from build123d import *

# Parameters (mm, degrees)
F0_W      = 858
F0_H      = 170
F1_DEPTH  = 19
F2_W      = 19
F2_H      = 170
F3_DEPTH  = 590
F4_W      = 19
F4_H      = 170
F5_DEPTH  = 824
F6_W      = 820
F6_H      = 5
F7_DEPTH  = 8
F8_W      = 820
F8_H      = 5
F9_DEPTH  = 8
F11_DEPTH = 8
F13_DEPTH = 8
F14_R     = 2
F15_DEPTH = 19


with BuildPart() as f1:
    # F0 (on Front) → F1 (new body)
    with BuildSketch(Plane.XZ):
        with Locations((-9.432035, -4.196442)):
            Rectangle(F0_W, F0_H)
    extrude(amount=F1_DEPTH)

    # F2 (on face) → F3 (join)
    with BuildSketch(Plane(origin=(0, 0, 0), x_dir=(-1, 0, 0), z_dir=(0, 1, 0))):
        with Locations((-410.067965, -4.196442)):
            Rectangle(F2_W, F2_H)
        with Locations((428.932035, -4.196442)):
            Rectangle(F2_W, F2_H)
    extrude(amount=F3_DEPTH)

    # F4 (on face) → F5 (join)
    with BuildSketch(Plane(origin=(400.567965, 0, 0), x_dir=(0, -1, 0), z_dir=(-1, 0, 0))):
        with Locations((-580.5, -4.196442)):
            Rectangle(F4_W, F4_H)
    extrude(amount=F5_DEPTH)

    # F6 (on face) → F7 (cut)
    with BuildSketch(Plane.XZ.offset(-571)):
        with Locations((-9.432035, -81.696442)):
            Rectangle(F6_W, F6_H)
    extrude(amount=-F7_DEPTH, mode=Mode.SUBTRACT)

    # F8 (on face) → F9 (cut)
    with BuildSketch(Plane(origin=(0, 0, 0), x_dir=(-1, 0, 0), z_dir=(0, 1, 0))):
        with Locations((9.432035, -81.696442)):
            Rectangle(F8_W, F8_H)
    extrude(amount=-F9_DEPTH, mode=Mode.SUBTRACT)

    # F10 (on face) → F11 (cut)
    with BuildSketch(Plane.YZ.offset(-419.432035)):
        Polygon((0, -79.196442), (-8, -79.196442), (-8, -84.196442), (0, -84.196442), (571, -84.196442), (579, -84.196442), (579, -79.196442), (571, -79.196442), align=None)
    extrude(amount=-F11_DEPTH, mode=Mode.SUBTRACT)

    # F12 (on face) → F13 (cut)
    with BuildSketch(Plane(origin=(400.567965, 0, 0), x_dir=(0, -1, 0), z_dir=(-1, 0, 0))):
        Polygon((8, -84.196442), (8, -79.196442), (0, -79.196442), (-571, -79.196442), (-579, -79.196442), (-579, -84.196442), (-571, -84.196442), (0, -84.196442), align=None)
    extrude(amount=-F13_DEPTH, mode=Mode.SUBTRACT)

    # F14 (on face) → F15 (cut)
    with BuildSketch(Plane.XZ.offset(19)):
        Circle(F14_R)
    extrude(amount=-F15_DEPTH, mode=Mode.SUBTRACT)


solid = f1.part
Model file for the job. Use its own axes, mm. A direction names the side the tool comes from. Coordinates: 2 decimals unless noted, no trailing zeros. Write each loop counter-clockwise with the first axis right and the second up, starting at its lowest first coordinate (ties: lowest second). Pieces come first, ordered by that corner, then holes. Notation, with made-up numbers: (-20, -2.5) -> (-12, -2.5) arc R18 cw to (-12, 19.5) -> close; hole circle Ø8 at (67, 59). An arc over 180 degrees is marked (long way). One line per item, written item: value. Start each with the question number.
1) Slice it at B-B on x = -40. Write the cut outline in (y, z), then the cut area to 3 significant figures.
2) Probe probe 1 along Y at (x, z) = (-234, 69.5); probe 2 along Z at (x, y) = (0, -6); probe 3 along Z at (x, y) = (0, -14). List the from-to ranges inside material, lowest first.
3) Pull direction Y, two halves, no side cores. Call faces 3 (the face through (-438.432, 290, -5)), 4 (the face through (-3, 590, -5)), 5 (the face through (-419.432, 282, 0)), 6 (the face through (-4, 571, 0)): +Y half, -Y half, draft (parallel to the pull), parting line (faces both ways), or undercut.
4) Flat gauge pin, fed straight in: pin 1 Ø4.5 at (x, z) = (0, 0) entering from -Y. Where does the tip first touch, or does it go through?
5) Which spindle directions (+Z, -Z, +X, -X, +Y, -Y) get a long thin tool onto all of the face, cutting with end or side? Do faces 1 (the face through (-15, -19, -3)), 2 (the face through (-15, 0, 2)). Say none if no direction does.
6) Slice it at A-A on y = 551. Write the cut outline in (x, z).
7) Slice it at C-C on z = 42. Write the cut outline in (x, y).
Answers follow:
1. outline: (-19, -89.2) -> (0, -89.2) -> (0, -84.2) -> (-8, -84.2) -> (-8, -79.2) -> (0, -79.2) -> (0, 80.8) -> (-19, 80.8) -> close; (571, -89.2) -> (590, -89.2) -> (590, 80.8) -> (571, 80.8) -> (571, -79.2) -> (579, -79.2) -> (579, -84.2) -> (571, -84.2) -> close
1. area: 6,380 mm2
2. probe 1: -19 to 0, 571 to 590
2. probe 2: -89.2 to -84.2, -79.2 to -2, 2 to 80.8
2. probe 3: -89.2 to -2, 2 to 80.8
3. face 3: draft
3. face 4: +Y half
3. face 5: undercut
3. face 6: undercut
4. pin 1: y = -19
5. face 1: +Z, -Z, +X, -X, -Y
5. face 2: +Z, -Z
6. outline: (-438.43, -89.2) -> (-419.43, -89.2) -> (-419.43, -84.2) -> (-427.43, -84.2) -> (-427.43, -79.2) -> (-419.43, -79.2) -> (-419.43, 80.8) -> (-438.43, 80.8) -> close; (400.57, -89.2) -> (419.57, -89.2) -> (419.57, 80.8) -> (400.57, 80.8) -> (400.57, -79.2) -> (408.57, -79.2) -> (408.57, -84.2) -> (400.57, -84.2) -> close
7. outline: (-438.43, -19) -> (419.57, -19) -> (419.57, 590) -> (-438.43, 590) -> close; hole (-419.43, 0) -> (400.57, 0) -> (400.57, 571) -> (-419.43, 571) -> close
